Geometry: final body of the model. Coordinates: model frame, mm. A direction names the side the tool comes from. Round coordinates to 2 decimals unless told otherwise and drop trailing zeros. Write each loop counter-clockwise with the first axis right and the second up, starting at its lowest first coordinate (ties: lowest second). Pieces come first, ordered by that corner, then holes. Notation, with made-up numbers: (81, 7.25) - (114, 7.25) arc R20 cw to (114, 24.25) - close; hole circle Ø10 at (13.5, 42.25). An arc over 180 degrees is marked (long way). Use a Markdown table: item, result. Add a question column.
```python
from build123d import *

# Parameters (mm, degrees)
F0_W           = 22
F0_H           = 19
F1_DEPTH       = 3
F2_W           = 60
F2_H           = 3
F2_W_2         = 3
F2_H_2         = 19
F3_DEPTH       = 16
F5_D           = 4
F5_DEPTH       = 12
F5_CSINK_D     = 8
F5_CSINK_ANGLE = 90
F5_TIP         = 1.2017212381
F7_D           = 4
F7_DEPTH       = 12
F7_CSINK_D     = 8
F7_CSINK_ANGLE = 90
F7_TIP         = 1.2017212381
F9_D           = 4
F9_DEPTH       = 12
F9_CSINK_D     = 8
F9_CSINK_ANGLE = 90
F9_TIP         = 1.2017212381
F10_SIZE       = 0.75
F11_SIZE       = 0.75
F12_SIZE       = 0.75
F13_SIZE       = 0.75


with BuildPart() as f1:
    # F0 (on Top) → F1 (new body)
    with BuildSketch(Plane.XY):
        Polygon((0, 22), (0, 0), (19, 0), (41, 0), (60, 0), (60, 22), align=None)
        with Locations((30, -9.5)):
            Rectangle(F0_W, F0_H)
    extrude(amount=F1_DEPTH)

    # F2 (on face) → F3 (join)
    with BuildSketch(Plane.XY.offset(3)):
        with Locations((30, 20.5)):
            Rectangle(F2_W, F2_H)
        Polygon((0, 0), (19, 0), (22, 0), (22, 3), (0, 3), align=None)
        with Locations((20.5, -9.5)):
            Rectangle(F2_W_2, F2_H_2)
        with Locations((39.5, -9.5)):
            Rectangle(F2_W_2, F2_H_2)
        Polygon((38, 0), (41, 0), (60, 0), (60, 3), (38, 3), align=None)
    extrude(amount=F3_DEPTH)

    # F5
    with Locations(Plane.XZ):
        with Locations((50.5, 9.5)):
            CounterSinkHole(F5_D / 2, F5_CSINK_D / 2, depth=F5_DEPTH, counter_sink_angle=F5_CSINK_ANGLE)
            with Locations((0, 0, -(F5_DEPTH + F5_TIP / 2))):  # 118° drill point
                Cone(0, F5_D / 2, F5_TIP, mode=Mode.SUBTRACT)

    # F7
    with Locations(Plane.YZ.offset(41)):
        with Locations((-9.5, 9.5)):
            CounterSinkHole(F7_D / 2, F7_CSINK_D / 2, depth=F7_DEPTH, counter_sink_angle=F7_CSINK_ANGLE)
            with Locations((0, 0, -(F7_DEPTH + F7_TIP / 2))):  # 118° drill point
                Cone(0, F7_D / 2, F7_TIP, mode=Mode.SUBTRACT)

    # F9
    with Locations(Plane.XZ):
        with Locations((9.5, 9.5)):
            CounterSinkHole(F9_D / 2, F9_CSINK_D / 2, depth=F9_DEPTH, counter_sink_angle=F9_CSINK_ANGLE)
            with Locations((0, 0, -(F9_DEPTH + F9_TIP / 2))):  # 118° drill point
                Cone(0, F9_D / 2, F9_TIP, mode=Mode.SUBTRACT)

    # F10
    f10_edges = [f1.edges().sort_by_distance(p)[0] for p in [
        (60, 0, 9.5),
        (60, 1.5, 19),
        (60, 3, 11),
        (60, 11, 3),
        (60, 19, 11),
        (60, 20.5, 19),
        (60, 22, 9.5),
        (60, 11, 0),
        (19, -19, 9.5),
        (20.5, -19, 19),
        (22, -19, 11),
        (30, -19, 3),
        (38, -19, 11),
        (39.5, -19, 19),
        (41, -19, 9.5),
        (30, -19, 0),
        (0, 22, 9.5),
        (0, 20.5, 19),
        (0, 19, 11),
        (0, 11, 3),
        (0, 3, 11),
        (0, 1.5, 19),
        (0, 0, 9.5),
        (0, 11, 0),
    ]]
    chamfer(f10_edges, length=F10_SIZE)

    # F11
    f11_edges = [f1.edges().sort_by_distance(p)[0] for p in [
        (38, 3, 11),
        (22, 3, 11),
    ]]
    chamfer(f11_edges, length=F11_SIZE)

    # F12 (call 1 of 8: OpenCascade refuses the feature's edges together)
    f12_edges = [f1.edges().sort_by_distance(p)[0] for p in [
        (30, 22, 19),
    ]]
    chamfer(f12_edges, length=F12_SIZE)

    # F12#2 (call 2 of 8)
    f12_2_edges = [f1.edges().sort_by_distance(p)[0] for p in [
        (30, 19, 19),
    ]]
    chamfer(f12_2_edges, length=F12_SIZE)

    # F12#3 (call 3 of 8)
    f12_3_edges = [f1.edges().sort_by_distance(p)[0] for p in [
        (49, 3, 19),
    ]]
    chamfer(f12_3_edges, length=F12_SIZE)

    # F12#4 (call 4 of 8)
    f12_4_edges = [f1.edges().sort_by_distance(p)[0] for p in [
        (50.125, 0, 19),
        (41, -9.125, 19),
    ]]
    chamfer(f12_4_edges, length=F12_SIZE)

    # F12#5 (call 5 of 8)
    f12_5_edges = [f1.edges().sort_by_distance(p)[0] for p in [
        (38, -8, 19),
    ]]
    chamfer(f12_5_edges, length=F12_SIZE)

    # F12#6 (call 6 of 8)
    f12_6_edges = [f1.edges().sort_by_distance(p)[0] for p in [
        (22, -8, 19),
    ]]
    chamfer(f12_6_edges, length=F12_SIZE)

    # F12#7 (call 7 of 8)
    f12_7_edges = [f1.edges().sort_by_distance(p)[0] for p in [
        (19, -9.125, 19),
        (9.875, 0, 19),
    ]]
    chamfer(f12_7_edges, length=F12_SIZE)

    # F12#8 (call 8 of 8)
    f12_8_edges = [f1.edges().sort_by_distance(p)[0] for p in [
        (11, 3, 19),
    ]]
    chamfer(f12_8_edges, length=F12_SIZE)

    # F13
    f13_edges = [f1.edges().sort_by_distance(p)[0] for p in [
        (9.875, 0, 0),
        (19, -9.125, 0),
        (41, -9.125, 0),
        (50.125, 0, 0),
        (30, 22, 0),
    ]]
    chamfer(f13_edges, length=F13_SIZE)


solid = f1.part
```
1) Section C-C, the plane x = 9.5. Return the cut outline in (y, z).
2) Material intervals for L1, parallel to Y at x = 38.75, z = 9.5; L2, parallel to Y at x = 5.5, z = 7.75; L3, parallel to X at y = -14, z = 15.5, sorted ascending. Write a range as from..to.
3) Pin query (flat end, axial travel): P1, Ø5, axis at x = 50.5, z = 9.5, coming from the -Y side; P2, Ø3.5, axis at y = -9.5, z = 9.5, coming from the -X side; P3, Ø4.5, axis at x = 9.5, z = 9.5, coming from the -Y side. Return the tip coordinate at first contact, or that it passes through.
4) Draft query along Z for faces 6 (the flat face through (19, -9, 9)), 7 (the flat face through (40, -3, 19)), 8 (the cylindrical face through (38.493, -9.24, 11.483)). Return one class per face: released by +Z, released by -Z, zero draft, split by the parting line, or undercut.
5) Section A-A, the plane y = -9.5. Return the cut outline in (x, z), then the cut area to 3 significant figures.
6) Section B-B, the plane z = 4.75. State how many separate pieces and enclosed holes the cut face has, then the cut area to 3 significant figures.
7) Section D-D, the plane y = 10.5. Return the cut outline in (x, z), then the cut area to 3 significant figures.
8) Set-up query: faces 1 (the flat face through (41, -9, 5)), 2 (the flat face through (38, -8, 12)), 3 (the flat face through (30, 5, 3)), 4 (the cylindrical face through (9.76, 2.507, 11.483)), 5 (the flat face through (49, 3, 12)). Return all of +Z, -Z, +X, -X, +Y, -Y with unobstructed straight access to the full face (end or side cutting, diameter ignored); none if empty.
Output values:
| question | item | result |
|---|---|---|
| 1 | outline | (0, 0.75) - (0.75, 0) - (21.25, 0) - (22, 0.75) - (22, 18.25) - (21.25, 19) - (19.75, 19) - (19, 18.25) - (19, 3) - (3, 3) - (3, 7.5) - (2, 7.5) - (0, 5.5) - close; (0, 13.5) - (2, 11.5) - (3, 11.5) - (3, 18.25) - (2.25, 19) - (0.75, 19) - (0, 18.25) - close |
| 2 | L1 | y = -19..-11.5, -7.5..3, 19..22 |
| 2 | L2 | y = 0..3, 19..22 |
| 2 | L3 | x = 19..22, 38..41 |
| 3 | P1 | stops at y = 1.5 |
| 3 | P2 | stops at x = 19 |
| 3 | P3 | stops at y = 1.75 |
| 4 | face 6 | zero draft |
| 4 | face 7 | released by +Z |
| 4 | face 8 | undercut |
| 5 | outline | (19, 0.75) - (19.75, 0) - (40.25, 0) - (41, 0.75) - (41, 5.5) - (39, 7.5) - (38, 7.5) - (38, 3) - (22, 3) - (22, 18.25) - (21.25, 19) - (19.75, 19) - (19, 18.25) - close; (38, 11.5) - (39, 11.5) - (41, 13.5) - (41, 18.25) - (40.25, 19) - (38.75, 19) - (38, 18.25) - close |
| 5 | area | 144 mm^2 |
| 6 | separate pieces | 3 |
| 6 | enclosed holes | 0 |
| 6 | area | 422 mm^2 |
| 7 | outline | (0, 0.75) - (0.75, 0) - (59.25, 0) - (60, 0.75) - (60, 2.25) - (59.25, 3) - (0.75, 3) - (0, 2.25) - close |
| 7 | area | 179 mm^2 |
| 8 | face 1 | +Z, -Z, +X, -Y |
| 8 | face 2 | +Z, -Y |
| 8 | face 3 | +Z |
| 8 | face 4 | -Y |
| 8 | face 5 | +Z, +X, -X |
